Autodesk Inventor part; units mm, degrees
ref_plane "YZ Plane" through (0, 0, 0) normal (1, 0, 0) x (0, 1, 0)
ref_plane "XZ Plane" through (0, 0, 0) normal (0, 1, 0) x (-1, 0, 0)
ref_plane "XY Plane" through (0, 0, 0) normal (0, 0, 1) x (1, 0, 0)
sketch "Sketch2" plane through (0, 0, 0) normal (0, 0, 1) x (1, 0, 0)
  circle A0 centre (-65.2715, -43.4254) radius 46.99
  line L0 (-19.2425, -52.8797) -> (108.4608, 36.9121)
  line L1 (108.4608, 36.9121) -> (68.0869, 93.186)
  line L2 (68.0869, 93.186) -> (-55.5981, 2.5581)
  circle A1 centre (100.0461, 41.8214) radius 2.54
  circle A2 centre (66.5651, 84.6941) radius 2.54
  circle A3 centre (-65.5862, -43.4643) radius 5.08
  circle A4 centre (67.9257, 44.5075) radius 5.08
  circle A5 centre (29.8863, 20.6511) radius 2.54
  circle A6 centre (10.4927, 4.2484) radius 2.54
  circle A7 centre (-18.5977, -20.3557) radius 2.54
  circle A8 centre (-28.2944, -28.557) radius 2.54
  point P0 (0, 0)
  dimension "d45" = 93.98
  dimension "d46" = 127.7033
  dimension "d47" = 153.3343
  dimension "d48" = 5.08
  dimension "d49" = 5.08
  dimension "d50" = 10.16
  dimension "d51" = 10.16
  dimension "d52" = 5.08
  dimension "d53" = 5.08
  dimension "d54" = 5.08
  dimension "d55" = 5.08
extrude "Extrusion2" add sketch "Sketch2" along normal blind 1.5875
fillet "Fillet2" radius 3.175 4 edges at (-55.5981, 2.5581, 0.7937) (68.0869, 93.186, 0.7937) (108.4608, 36.9121, 0.7937) (-19.2425, -52.8797, 0.7937)
properties part number "Intake poly"
Read the model definition and answer for the solid it produces. Units are mm, in the model's axes. Coordinates: 2 decimals unless noted, no trailing zeros. Write each loop counter-clockwise with the first axis right and the second up, starting at its lowest first coordinate (ties: lowest second). Pieces come first, ordered by that corner, then holes. Notation, with made-up numbers: (72, 76) -> (84, 76) arc R11 ccw to (84, 85) -> close; hole circle Ø2 at (24.5, 60). An arc over 180 degrees is marked (long way). Return JSON: item names as keys, results as strings.
1. Find the intervals of material crossed by line 1 along Y through (x, z) = (65, 0.6); line 2 along X through (y, z) = (47, 1.5); line 3 along X through (y, z) = (-47, 0.7), in increasing order. Write a range as from..to.
Found:
{"line 1": "6.35..40.35, 48.66..82.69, 86.69..90.92", "line 2": "5.05..63.5, 72.35..101.22", "line 3": "-112.13..-69.23, -61.94..-10.88"}
2. A cutting plane is placed at C-C (x = -80.5). Determine the outline of the cut face in (y, z).
Found:
{"outline": "(-87.88, 0) -> (1.03, 0) -> (1.03, 1.59) -> (-87.88, 1.59) -> close"}
3. A cutting plane is placed at A-A (z = 1.1). Give the number of separate pieces and of enclosed holes in the cut face, and give its area (3 significant figures).
Found:
{"separate pieces": "1", "enclosed holes": "8", "area": "16,500 mm2"}
4. A cutting plane is placed at B-B (y = -33.5). Determine the outline of the cut face in (x, z), and give its area (3 significant figures).
Found:
{"outline": "(-111.2, 0) -> (8.32, 0) -> (8.32, 1.59) -> (-111.2, 1.59) -> close", "area": "190 mm2"}
5. Determine the mould class of faces 1 (the face through (-4, 2, 1.588)), 2 (the face through (29.34, 23.13, 0.78)), 3 (the face through (42.935, -9.161, 0.783)) for opening direction X: pulls with the +X half, pulls with the -X half, needs draft (parallel to the pull), parting line crosses it, or undercut.
Found:
{"face 1": "needs draft", "face 2": "undercut", "face 3": "pulls with the +X half"}
